```python
from build123d import *

# Parameters (mm, degrees)
SZKIC1_R                    = 6
DODANIE_WYCI_GNI_CIE1_DEPTH = 64
SZKIC2_OUTSIDE_W            = 27.242
SZKIC2_OUTSIDE_H            = 27.242
SZKIC2_OUTSIDE_R            = 4.9
WYTNIJ_WYCI_GNI_CIE1_DEPTH  = 47
SZKIC3_OUTSIDE_W            = 27.242
SZKIC3_OUTSIDE_H            = 27.242
SZKIC3_OUTSIDE_R            = 4.5
WYTNIJ_WYCI_GNI_CIE2_DEPTH  = 16.5


with BuildPart() as part:
    # Szkic1 → Dodanie-wyciągnięcie1 (new body)
    with BuildSketch(Plane.XY):
        Circle(SZKIC1_R)
    extrude(amount=DODANIE_WYCI_GNI_CIE1_DEPTH)

    # Szkic2 outside → Wytnij-wyciągnięcie1 (cut)
    with BuildSketch(Plane(origin=(0, 0, 0), x_dir=(-1, 0, 0), z_dir=(0, 0, -1))):
        Rectangle(SZKIC2_OUTSIDE_W, SZKIC2_OUTSIDE_H)
        Circle(SZKIC2_OUTSIDE_R, mode=Mode.SUBTRACT)
    extrude(amount=-WYTNIJ_WYCI_GNI_CIE1_DEPTH, mode=Mode.SUBTRACT)

    # Szkic3 outside → Wytnij-wyciągnięcie2 (cut)
    with BuildSketch(Plane.XY.offset(64)):
        Rectangle(SZKIC3_OUTSIDE_W, SZKIC3_OUTSIDE_H)
        Circle(SZKIC3_OUTSIDE_R, mode=Mode.SUBTRACT)
    extrude(amount=-WYTNIJ_WYCI_GNI_CIE2_DEPTH, mode=Mode.SUBTRACT)


solid = part.part
```
Input: part model. Units: mm. Frame: model coordinates. A direction names the side the tool comes from. Coordinates: 2 decimals unless noted, no trailing zeros. Write each loop counter-clockwise with the first axis right and the second up, starting at its lowest first coordinate (ties: lowest second). Pieces come first, ordered by that corner, then holes.
1) Section D-D on z = 46. Output: boundary loops of the cut face in (x, y).
2) Section A-A on x = 0. Output: boundary loops of the cut face in (y, z), and give its area (3 significant figures).
3) Pin query (flat end, axial travel): pin 1 Ø1.5 at (y, z) = (0.5, 22.5) entering from +X; pin 2 Ø4 at (y, z) = (-4, 56) entering from -X. Return the tip coordinate at first contact, or that it passes through.
4) Set-up query: faces 1 (the cylindrical face through (1.062, -4.783, 23.171)), 2 (the flat face through (-1.4, 4.5, 47.5)), 3 (the flat face through (0, 0, 0)). Return all of +Z, -Z, +X, -X, +Y, -Y with unobstructed straight access to the full face (end or side cutting, diameter ignored); none if empty.
5) Material intervals for line 1 along Y through (x, z) = (-0.25, 32); line 2 along Z through (x, y) = (1.5, -5); line 3 along X through (y, z) = (0.25, 61.5), sorted ascending.
6) Section C-C on z = 58. Output: boundary loops of the cut face in (x, y), and give its area (3 significant figures).
Check result:
1. outline: circle Ø9.8 at (0, 0)
2. outline: (-6, 47) - (-4.9, 47) - (-4.9, 0) - (4.9, 0) - (4.9, 47) - (6, 47) - (6, 47.5) - (4.5, 47.5) - (4.5, 64) - (-4.5, 64) - (-4.5, 47.5) - (-6, 47.5) - close
2. area: 615 mm2
3. pin 1: stops at x = 4.9
3. pin 2: stops at x = -4.03
4. face 1: -Z
4. face 2: +Z
4. face 3: -Z, +X, -X, +Y, -Y
5. line 1: y = -4.89 to 4.89
5. line 2: z = 47 to 47.5
5. line 3: x = -4.49 to 4.49
6. outline: circle Ø9 at (0, 0)
6. area: 63.6 mm2
